Build history of the part. All positions in model axes, mm. Face numbers are marked on the shaded views. A direction names the side the tool comes from. Give positions to 0.01 mm unless a question says otherwise; leave off trailing zeros. Order: outer loops, then holes, each group sorted by start corner. A loop starts at its lowest first (then second) coordinate and runs counter-clockwise, first axis right, second up. Notation, with made-up numbers: (20.5, -14) - (28.5, -14) arc R23 ccw to (28.5, 12) - close; hole circle Ø6 at (31, 44). An arc over 180 degrees is marked (long way). Write each question's results on one line, items separated by ' | '. Start each with the question number.
from build123d import *

# Parameters (mm, degrees)
SKETCH1_W           = 150
SKETCH1_H           = 36
BOSS_EXTRUDE1_DEPTH = 1.5
SKETCH2_W           = 150
SKETCH2_H           = 36
SKETCH2_W_2         = 132.5
SKETCH2_H_2         = 32
BOSS_EXTRUDE2_DEPTH = 15
SKETCH3_W           = 12
SKETCH3_H           = 9.5
CUT_EXTRUDE1_DEPTH  = 8.75
SKETCH4_W           = 33.5
SKETCH4_H           = 13
CUT_EXTRUDE2_DEPTH  = 2
BOSS_EXTRUDE4_DEPTH = 16.5
FILLET1_R           = 10
SKETCH5_R           = 1.375
CUT_EXTRUDE3_DEPTH  = 7.5
SKETCH8_W           = 36.55
SKETCH8_H           = 3.25
BOSS_EXTRUDE3_DEPTH = 2
FILLET2_R           = 5
FILLET3_R           = 1
CHAMFER1_SIZE       = 1
SKETCH10_W          = 113.75
SKETCH10_H          = 3.25
CUT_EXTRUDE4_DEPTH  = 0.25


with BuildPart() as part:
    # Sketch1 → Boss-Extrude1 (new body)
    with BuildSketch(Plane(origin=(0, 0, 0), x_dir=(1, 0, 0), z_dir=(0, 1, 0))):
        with Locations((-63, 12.75)):
            Rectangle(SKETCH1_W, SKETCH1_H)
        with BuildLine():
            Line((0, 0), (-110.5, 0))
            ThreePointArc((-110.5, 0), (-121.460155108, 4.539844892), (-126, 15.5))
            Line((-126, 15.5), (-126, 25.5))
            Line((-126, 25.5), (-11.5, 25.5))
            ThreePointArc((-11.5, 25.5), (-3.368272016, 22.131727984), (0, 14))
            Line((0, 14), (0, 0))
        make_face(mode=Mode.SUBTRACT)
    extrude(amount=BOSS_EXTRUDE1_DEPTH)

    # Sketch2 → Boss-Extrude2 (add)
    with BuildSketch(Plane.XZ):
        with Locations((-63, -12.75)):
            Rectangle(SKETCH2_W, SKETCH2_H)
        with Locations((-63, -12.75)):
            Rectangle(SKETCH2_W_2, SKETCH2_H_2, mode=Mode.SUBTRACT)
    extrude(amount=BOSS_EXTRUDE2_DEPTH)

    # Sketch3 → Cut-Extrude1 (cut)
    with BuildSketch(Plane.ZY.offset(-12)):
        with Locations((-2.75, -10.25)):
            Rectangle(SKETCH3_W, SKETCH3_H)
    extrude(amount=CUT_EXTRUDE1_DEPTH, mode=Mode.SUBTRACT)

    # Sketch4 → Cut-Extrude2 (cut)
    with BuildSketch(Plane.XY.offset(-30.75)):
        with Locations((-106.2, -8.5)):
            Rectangle(SKETCH4_W, SKETCH4_H)
    extrude(amount=CUT_EXTRUDE2_DEPTH, mode=Mode.SUBTRACT)

    # Sketch9 → Boss-Extrude4 (add)
    with BuildSketch(Plane(origin=(0, 1.5, 0), x_dir=(1, 0, 0), z_dir=(0, 1, 0))):
        with BuildLine():
            Line((-68, 33.25), (-68, 30.75))
            Line((-68, 30.75), (-58, 30.75))
            Line((-58, 30.75), (-58, 33.25))
            ThreePointArc((-58, 33.25), (-63, 38.25), (-68, 33.25))
        make_face()
        with BuildLine():
            Line((-58, -7.75), (-58, -5.25))
            Line((-58, -5.25), (-68, -5.25))
            Line((-68, -5.25), (-68, -7.75))
            ThreePointArc((-68, -7.75), (-63, -12.75), (-58, -7.75))
        make_face()
    extrude(amount=-BOSS_EXTRUDE4_DEPTH)

    # Fillet1
    fillet1_edges = [part.edges().sort_by_distance(p)[0] for p in [
        (12, -6.75, -30.75),
        (-138, -6.75, 5.25),
    ]]
    fillet(fillet1_edges, radius=FILLET1_R)

    # Sketch5 → Cut-Extrude3 (cut)
    with BuildSketch(Plane(origin=(0, -15, 0), x_dir=(1, 0, 0), z_dir=(0, 1, 0))):
        with Locations(Location((7.5, 21.5, 0), (0, 0, 270))):
            Circle(SKETCH5_R)
        with Locations((7.5, 4)):
            Circle(SKETCH5_R)
        with Locations(Location((-133.5, 4, 0), (0, 0, 270))):
            Circle(SKETCH5_R)
        with Locations(Location((-133.5, 21.5, 0), (0, 0, 270))):
            Circle(SKETCH5_R)
        with Locations(Location((-63, -7.75, 0), (0, 0, 270))):
            Circle(SKETCH5_R)
        with Locations(Location((-63, 33.25, 0), (0, 0, 270))):
            Circle(SKETCH5_R)
    extrude(amount=CUT_EXTRUDE3_DEPTH, mode=Mode.SUBTRACT)

    # Sketch8 → Boss-Extrude3 (add)
    with BuildSketch(Plane.XZ):
        with Locations((-107.725, -27.125)):
            Rectangle(SKETCH8_W, SKETCH8_H)
    extrude(amount=BOSS_EXTRUDE3_DEPTH)

    # Fillet2
    # the kernel refuses this fillet: 5 mm, written as the material it adds along each edge
    with BuildSketch(Plane(origin=(-58, 1.5, -30.75), x_dir=(1, 0, 0), z_dir=(0, -1, 0)), Plane(origin=(-68, 1.5, 5.25), x_dir=(-1, 0, 0), z_dir=(0, -1, 0))) as fillet2_piece_1:
        with BuildLine():
            CenterArc((4.682458366, -5), FILLET2_R, 90, 75.522487814)
            Line((-0.158770817, -3.75), (-0.642893736, -3.625))
            ThreePointArc((-0.642893736, -3.625), (-0.5, -2.5), (-0.5, 0))
            Line((-0.5, 0), (0, 0.5))
            Line((0, 0.5), (4.682458366, 0.5))
            Line((4.682458366, 0.5), (4.682458366, 0))
        make_face()
    extrude(amount=16.5)
    with BuildSketch(Plane(origin=(-68, 1.5, -30.75), x_dir=(-1, 0, 0), z_dir=(0, -1, 0))) as fillet2_piece_2:
        with BuildLine():
            CenterArc((4.682458366, 5), FILLET2_R, 194.477512186, 75.522487814)
            Line((-0.158770817, 3.75), (-0.642893736, 3.625))
            ThreePointArc((-0.642893736, 3.625), (-0.5, 2.5), (-0.5, 0))
            Line((-0.5, 0), (0, -0.5))
            Line((0, -0.5), (4.682458366, -0.5))
            Line((4.682458366, -0.5), (4.682458366, 0))
        make_face()
    extrude(amount=16.5)
    with BuildSketch(Plane(origin=(-58, 1.5, 5.25), x_dir=(-0.0423009875968097, 0, 0.9991049126334705), z_dir=(0, -1, 0))) as fillet2_piece_3:
        with BuildLine():
            CenterArc((4.79745195, -4.889772094), FILLET2_R, 102.053120737, 75.522487814)
            Line((-0.198072613, -4.678267156), (-0.69762507, -4.657116662))
            Line((-0.69762507, -4.657116662), (-0.499552456, 0.021150494))
            Line((-0.499552456, 0.021150494), (0.021150494, 0.499552456))
            ThreePointArc((0.021150494, 0.499552456), (2.518912775, 0.393799987), (3.648950348, 0.488977209))
            Line((3.648950348, 0.488977209), (3.753359585, 0))
        make_face()
    extrude(amount=16.5)
    # the kernel refuses this fillet: 5 mm, written as the material it takes off along each edge

    # Fillet3
    fillet3_edges = [part.edges().sort_by_distance(p)[0] for p in [
        (-25.658770817, 1.5, -30.75),
        (-100.341229183, 1.5, 5.25),
        (-135.071067812, 1.5, 2.321067812),
        (9.071067812, 1.5, -27.821067812),
        (12, 1.5, -7.75),
        (-63, 1.5, 12.75),
        (-20.658770817, 1.5, 5.25),
        (-63, 1.5, -38.25),
        (-105.341229183, 1.5, -30.75),
        (-56.379403813, 1.5, 6.297152925),
        (-69.620596187, 1.5, 6.297152925),
        (-56.379403813, 1.5, -31.797152925),
        (-69.620596187, 1.5, -31.797152925),
        (-138, 1.5, -17.75),
        (-138, -6.75, -30.75),
        (12, -6.75, 5.25),
    ]]
    fillet(fillet3_edges, radius=FILLET3_R)

    # Chamfer1
    chamfer1_edges = [part.edges().sort_by_distance(p)[0] for p in [
        (-63, -15, -34.625),
        (-133.5, -15, -5.375),
        (-133.5, -15, -22.875),
        (-63, -15, 6.375),
        (7.5, -15, -22.875),
    ]]
    chamfer(chamfer1_edges, length=CHAMFER1_SIZE)

    # Sketch10 → Cut-Extrude4 (cut)
    with BuildSketch(Plane.XZ):
        with Locations((-53.625, 1.625)):
            Rectangle(SKETCH10_W, SKETCH10_H)
    extrude(amount=-CUT_EXTRUDE4_DEPTH, mode=Mode.SUBTRACT)


solid = part.part
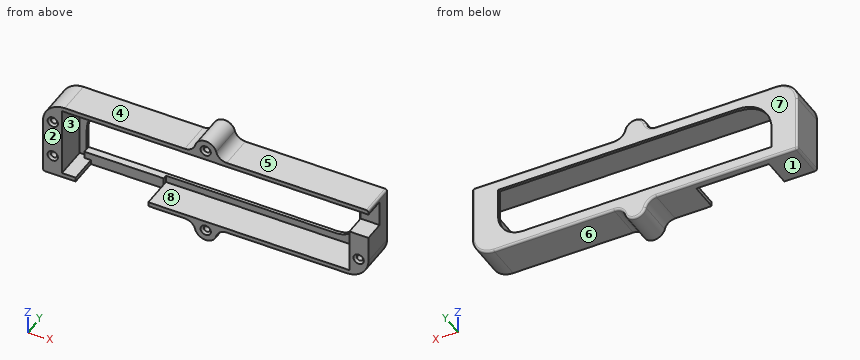
Item 1: Cut at B-B, the plane x = -63. List the corners of the cut face in (y, z) (3 decimals), then the cut area to 3 significant figures.
Item 2: Two-plate mould, pull along Z, no slides. Class the marked faces 6, 7 and 8: +Z half, -Z half, draft (parallel to the pull), parting line (faces both ways), or undercut.
Item 3: Probe line 1 along X through (y, z) = (-6.75, -11); line 2 along Z through (x, y) = (-87.5, -11.5); line 3 along X through (y, z) = (-10.5, -4) (3 decimals). List the from-to ranges inside material, lowest first. Write a range as from..to.
Item 4: Cut at C-C, the plane z = -10.5. List the corners of the cut face in (x, y), then the cut area to 3 significant figures.
Item 5: Cut at A-A, the plane y = -12.5. Count the separate pieces of the cut face and the enclosed holes in it, then the cut area to 3 significant figures.
Item 6: Flat gauge pins, fed straight in: pin 1 Ø6 at (x, z) = (-105, -27.5) entering from -Y; pin 2 Ø1 at (x, y) = (-45, -5) entering from +Z; pin 3 Ø2 at (x, z) = (-12.5, 7) entering from -Y; pin 4 Ø3 at (x, y) = (-76.5, 0) entering from +Z. Where does each tip first touch, or does it go through?
Item 7: Cut at D-D, the plane x = -81. List the corners of the cut face in (y, z).
Item 8: Which spindle directions (+Z, -Z, +X, -X, +Y, -Y) get a long thin tool onto all of the face, cutting with end or side? Do the marked faces 1, 2, 3, 4 and 5. Say none if no direction does.
Values found:
1) outline: (-15, -38.25) - (0.5, -38.25) arc R1 ccw to (1.5, -37.25) - (1.5, -25.5) - (0, -25.5) - (0, -28.75) - (-15, -28.75) - (-15, -30.875) - (-14, -31.875) - (-7.5, -31.875) - (-7.5, -34.625) - (-14, -34.625) - (-15, -35.625) - close; (-15, 3.25) - (0.25, 3.25) - (0.25, 0) - (1.5, 0) - (1.5, 11.75) arc R1 ccw to (0.5, 12.75) - (-15, 12.75) - (-15, 10.125) - (-14, 9.125) - (-7.5, 9.125) - (-7.5, 6.375) - (-14, 6.375) - (-15, 5.375) - close | area: 279 mm2
2) face 6: -Z half | face 7: draft | face 8: undercut
3) line 1: x = -138..-129.25, 3.25..12 | line 2: z = -30.75..-28.75, 3.25..5.25 | line 3: x = -137.972..-134.875, -132.125..-129.25
4) outline: (-138, -15) - (-129.25, -15) - (-129.25, 0) - (-125.17, 0) - (-125.17, 1.5) - (-137, 1.5) arc R1 ccw to (-138, 0.5) - close; (0, 0) - (3.25, 0) - (3.25, -15) - (12, -15) - (12, 0.5) arc R1 ccw to (11, 1.5) - (0, 1.5) - close | area: 299 mm2
5) separate pieces: 2 | enclosed holes: 5 | area: 1,060 mm2
6) pin 1: stops at y = -2 | pin 2: stops at z = 5.25 | pin 3: passes through | pin 4: stops at z = 5.25
7) outline: (-15, -30.75) - (0.5, -30.75) arc R1 ccw to (1.5, -29.75) - (1.5, -25.5) - (0, -25.5) - (0, -28.75) - (-15, -28.75) - close; (-15, 3.25) - (0.25, 3.25) - (0.25, 0) - (1.5, 0) - (1.5, 4.25) arc R1 ccw to (0.5, 5.25) - (-15, 5.25) - close
8) face 1: -Z, -X, +Y, -Y | face 2: +Z, -Z, +X, -X, -Y | face 3: -Y | face 4: +Z, -X, +Y, -Y | face 5: +Z, +X, +Y, -Y
